```python
from build123d import *

# Parameters (mm, degrees)
SKETCH2_R = 0.4


with BuildPart() as part:
    # Sweep1: sweep along a path in Sketch1
    with BuildLine(Plane(origin=(0, 0, 0), x_dir=(1, 0, 0), z_dir=(0, 1, 0))) as sweep1_path:
        Line((0, 0), (3, 0))
        Line((3, 0), (3, 3))
        Line((3, 3), (28, 3))
        Line((28, 3), (28, 13))
        Line((28, 13), (31, 13))
    # Sketch2 → Sweep1 (sweep)
    with BuildSketch(Plane(origin=(0, 0, 0), x_dir=(0, 0, -1), z_dir=(1, 0, 0))):
        Circle(SKETCH2_R)
    sweep(path=sweep1_path.line, transition=Transition.RIGHT)


solid = part.part
```
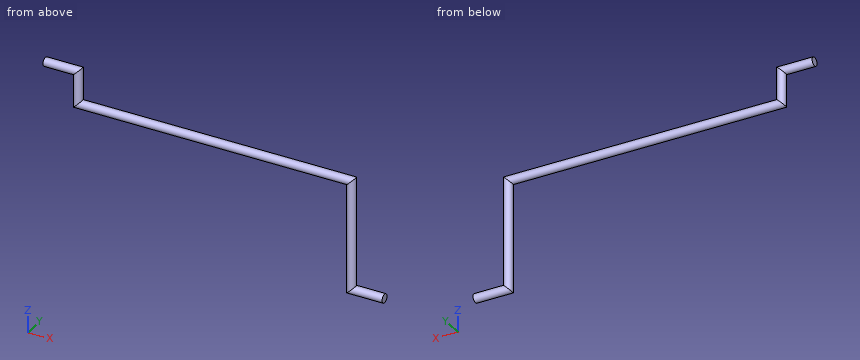
Work out the finished part from the listing and answer in its coordinate system (mm). Round coordinates to 2 decimals unless told otherwise and drop trailing zeros. Write each loop counter-clockwise with the first axis right and the second up, starting at its lowest first coordinate (ties: lowest second). Pieces come first, ordered by that corner, then holes. Notation, with made-up numbers: (29.5, 9.5) -> (83.5, 9.5) arc R23 ccw to (83.5, 40.5) -> close; hole circle Ø7 at (59.5, -10). An arc over 180 degrees is marked (long way). Write each question's results on one line, items separated by ' | '.
Q1. Section D-D, the plane x = 3 is taken. Write down the section's boundary in (y, z).
Data:
outline: (-0.4, -3) arc R0.4 ccw to (0.4, -3) -> (0.4, 0) arc R0.4 ccw to (-0.4, 0) -> close
Q2. Section A-A, the plane y = 0 is taken. Write down the section's boundary in (x, z).
Data:
outline: (0, -0.4) -> (2.6, -0.4) -> (2.6, -3.4) -> (27.6, -3.4) -> (27.6, -13.4) -> (31, -13.4) -> (31, -12.6) -> (28.4, -12.6) -> (28.4, -2.6) -> (3.4, -2.6) -> (3.4, 0.4) -> (0, 0.4) -> close
Q3. A flat-ended cylindrical pin translates along its axis: P1, Ø8, axis at x = 7.5, z = -7.5, coming from the -Y side. Find the tip coordinate at first contact, or state that the pin passes through.
Data:
P1: through
Q4. Section C-C, the plane z = -4.25 is taken. Write down the section's boundary in (x, y).
Data:
outline: circle Ø0.8 at (28, 0)
Q5. Straight lines are drawn through the part: line 1 along X through (y, z) = (0.05, -3.75); line 2 along Z through (x, y) = (14, 0.05); line 3 along X through (y, z) = (0.25, -3.5). For each, find the intervals that lie inside material, in ascending order. Write a range as [from, to].
Data:
line 1: [27.6, 28.4] | line 2: [-3.4, -2.6] | line 3: [27.69, 28.31]
Q6. Section B-B, the plane x = 8 is taken. Write down the section's boundary in (y, z), then the cut area to 3 significant figures.
Data:
outline: circle Ø0.8 at (0, -3) | area: 0.503 mm^2
